Read the model definition and answer for the solid it produces. Units are mm, in the model's axes. A direction names the side the tool comes from. Coordinates: 2 decimals unless noted, no trailing zeros. Loops run counter-clockwise (first coordinate to the right, second up) from the corner with the lowest first, then second, coordinate; pieces in that order, holes last. Notation, with made-up numbers: (24.25, -34) - (77.25, -34) arc R36 ccw to (77.25, 5) - close; hole circle Ø11 at (31.25, -6). An arc over 180 degrees is marked (long way). Use CSV: the item, a comma, the result in double quotes.
```python
from build123d import *

# Parameters (mm, degrees)
BOSS_EXTRUDE1_DEPTH = 254


with BuildPart() as part:
    # Sketch1 → Boss-Extrude1 (new body)
    with BuildSketch(Plane(origin=(0, 0, 0), x_dir=(1, 0, 0), z_dir=(0, 1, 0))):
        with BuildLine():
            Line((0, 0), (149.5044, 0))
            Line((149.5044, 0), (149.5044, 6.0706))
            Line((149.5044, 6.0706), (149.5044, 31.4706))
            ThreePointArc((149.5044, 31.4706), (148.717, 32.258), (147.9296, 31.4706))
            Line((147.9296, 31.4706), (147.9296, 6.0706))
            Line((147.9296, 6.0706), (138.1252, 6.0706))
            Line((138.1252, 6.0706), (138.1252, 31.4706))
            ThreePointArc((138.1252, 31.4706), (137.3378, 32.258), (136.5504, 31.4706))
            Line((136.5504, 31.4706), (136.5504, 6.0706))
            Line((136.5504, 6.0706), (126.746, 6.0706))
            Line((126.746, 6.0706), (126.746, 31.4706))
            ThreePointArc((126.746, 31.4706), (125.9586, 32.258), (125.1712, 31.4706))
            Line((125.1712, 31.4706), (125.1712, 6.0706))
            Line((125.1712, 6.0706), (115.3668, 6.0706))
            Line((115.3668, 6.0706), (115.3668, 31.4706))
            ThreePointArc((115.3668, 31.4706), (114.5794, 32.258), (113.792, 31.4706))
            Line((113.792, 31.4706), (113.792, 6.0706))
            Line((113.792, 6.0706), (103.9876, 6.0706))
            Line((103.9876, 6.0706), (103.9876, 31.4706))
            ThreePointArc((103.9876, 31.4706), (103.2002, 32.258), (102.4128, 31.4706))
            Line((102.4128, 31.4706), (102.4128, 6.0706))
            Line((102.4128, 6.0706), (92.6084, 6.0706))
            Line((92.6084, 6.0706), (92.6084, 31.4706))
            ThreePointArc((92.6084, 31.4706), (91.821, 32.258), (91.0336, 31.4706))
            Line((91.0336, 31.4706), (91.0336, 6.0706))
            Line((91.0336, 6.0706), (81.2292, 6.0706))
            Line((81.2292, 6.0706), (81.2292, 31.4706))
            ThreePointArc((81.2292, 31.4706), (80.4418, 32.258), (79.6544, 31.4706))
            Line((79.6544, 31.4706), (79.6544, 6.0706))
            Line((79.6544, 6.0706), (69.85, 6.0706))
            Line((69.85, 6.0706), (69.85, 31.4706))
            ThreePointArc((69.85, 31.4706), (69.0626, 32.258), (68.2752, 31.4706))
            Line((68.2752, 31.4706), (68.2752, 6.0706))
            Line((68.2752, 6.0706), (58.4708, 6.0706))
            Line((58.4708, 6.0706), (58.4708, 31.4706))
            ThreePointArc((58.4708, 31.4706), (57.6834, 32.258), (56.896, 31.4706))
            Line((56.896, 31.4706), (56.896, 6.0706))
            Line((56.896, 6.0706), (47.0916, 6.0706))
            Line((47.0916, 6.0706), (47.0916, 31.4706))
            ThreePointArc((47.0916, 31.4706), (46.3042, 32.258), (45.5168, 31.4706))
            Line((45.5168, 31.4706), (45.5168, 6.0706))
            Line((45.5168, 6.0706), (35.7124, 6.0706))
            Line((35.7124, 6.0706), (35.7124, 31.4706))
            ThreePointArc((35.7124, 31.4706), (34.925, 32.258), (34.1376, 31.4706))
            Line((34.1376, 31.4706), (34.1376, 6.0706))
            Line((34.1376, 6.0706), (24.3332, 6.0706))
            Line((24.3332, 6.0706), (24.3332, 31.4706))
            ThreePointArc((24.3332, 31.4706), (23.5458, 32.258), (22.7584, 31.4706))
            Line((22.7584, 31.4706), (22.7584, 6.0706))
            Line((22.7584, 6.0706), (12.954, 6.0706))
            Line((12.954, 6.0706), (12.954, 31.4706))
            ThreePointArc((12.954, 31.4706), (12.1666, 32.258), (11.3792, 31.4706))
            Line((11.3792, 31.4706), (11.3792, 6.0706))
            Line((11.3792, 6.0706), (1.5748, 6.0706))
            Line((1.5748, 6.0706), (1.5748, 31.4706))
            ThreePointArc((1.5748, 31.4706), (0.7874, 32.258), (0, 31.4706))
            Line((0, 31.4706), (0, 0))
        make_face()
    extrude(amount=BOSS_EXTRUDE1_DEPTH)


solid = part.part
```
Q1. Given P1, Ø3, axis at x = 109.5, y = 119.5, coming from the -Z side; P2, Ø11, axis at x = 52, y = 103.5, coming from the -Z side; P3, Ø6, axis at x = 85.5, z = -14.5, coming from the -Y side, each flat-ended and moving along its own axis, determine where each tip first touches the part or whether it passes through.
Reported:
P1,"stops at z = -6.07"
P2,"stops at z = -32.24"
P3,"passes through"
Q2. The part is cut by section A-A on z = -9. Give the number of separate pieces and of enclosed holes in the cut face, and give its area (3 significant figures).
Reported:
separate pieces,"14"
enclosed holes,"0"
area,"5,600 mm²"
Q3. For a pull along X with two mould halves and no side action, classify faces 3 (the face through (41, 125, -6.071)), 4 (the face through (57.1, 254, -9.2)), 5 (the face through (0, 125, -16)) as +X half, -X half, draft (parallel to the pull), parting line (faces both ways), or undercut.
Reported:
face 3,"undercut"
face 4,"draft"
face 5,"-X half"
Q4. The part is cut by section B-B on x = 77. Determine the outline of the cut face in (y, z).
Reported:
outline,"(0, -6.07) - (254, -6.07) - (254, 0) - (0, 0) - close"
Q5. A tool of negligible diameter and unlimited length cuts with its end or side. For faces 1 (the face through (147.93, 125, -19)), 2 (the face through (74, 125, 0)), from which of +Z, -Z, +X, -X, +Y, -Y can it reach the whole face along a straight path? Write none if from no direction.
Reported:
face 1,"-Z, +Y, -Y"
face 2,"+Z, +X, -X, +Y, -Y"
Q6. Find the intervals of material crossed by probe 1 along Z at (x, y) = (102, 92); probe 2 along Z at (x, y) = (80.5, 29), in increasing order. Write a range as [from, to].
Reported:
probe 1,"z = [-6.07, 0]"
probe 2,"z = [-32.26, 0]"
